Autodesk Inventor part; units mm, degrees
ref_plane "Start Plane" through (0, 0, 0) normal (0, 0, 1) x (1, 0, 0)
ref_plane "End Plane" through (0, 0, 100) normal (0, 0, 1) x (1, 0, 0)
ref_plane "YZ Plane" through (0, 0, 0) normal (1, 0, 0) x (0, 1, 0)
ref_plane "Start Plane" through (0, 0, 0) normal (0, 0, 1) x (1, 0, 0)
ref_plane "End Plane" through (0, 0, 100) normal (0, 0, 1) x (1, 0, 0)
sketch "Sketch2" plane through (0, 0, 0) normal (0, 0, 1) x (1, 0, 0)
  circle A0 centre (0, 0) radius 2.5
  circle A1 centre (0, 0) radius 4.2 construction
  line L0 (10, -10) -> (-10, -10) construction
  line L1 (-10, -10) -> (-10, 10) construction
  line L2 (-10, 10) -> (10, 10) construction
  line L3 (10, 10) -> (10, -10) construction
  line L4 (10, -10) -> (-10, 10) construction
  line L5 (-10, -10) -> (10, 10) construction
  line L6 (-4.1658, 3.1759) -> (-7.7464, 6.7565)
  line L7 (-10, 8.8) -> (-10, 3.95)
  line L8 (-10, 3.95) -> (-9.6, 3.95)
  line L9 (-9.6, 3.95) -> (-9.6, 3.2)
  line L10 (-9.6, 3.2) -> (-8.6, 3.2)
  line L11 (-8.6, 3.2) -> (-8.6, 6.4029)
  line L12 (-10, 0) -> (0, 0) construction
  line L13 (-8.8, 10) -> (-3.95, 10)
  line L14 (-3.95, 10) -> (-3.95, 9.6)
  line L15 (-3.95, 9.6) -> (-3.2, 9.6)
  line L16 (-3.2, 9.6) -> (-3.2, 8.6)
  line L17 (-3.2, 8.6) -> (-6.4029, 8.6)
  arc A2 (-8.8, 10) -> (-10, 8.8) centre (-8.8, 8.8) ccw
  arc A3 (-6.4029, 8.6) -> (-6.7565, 7.7464) centre (-6.4029, 8.1) ccw
  arc A4 (-7.7464, 6.7565) -> (-8.6, 6.4029) centre (-8.1, 6.4029) ccw
  arc A5 (-3.8668, 1.6394) -> (-4.2, 0) centre (0, 0) ccw
  arc A6 (-3.8668, 1.6394) -> (-4.1658, 3.1759) centre (-5.1558, 2.1859) ccw
  line L18 (-3.1759, 4.1658) -> (-6.7565, 7.7464)
  arc A7 (0, 4.2) -> (-1.6394, 3.8668) centre (0, 0) ccw
  arc A8 (-3.1759, 4.1658) -> (-1.6394, 3.8668) centre (-2.1859, 5.1558) ccw
  line L19 (-3.2, -9.6) -> (-3.2, -8.6)
  line L20 (-3.2, -8.6) -> (-6.4029, -8.6)
  line L21 (-8.8, -10) -> (-3.95, -10)
  arc A9 (-1.6394, -3.8668) -> (-3.1759, -4.1658) centre (-2.1859, -5.1558) ccw
  line L22 (-3.1759, -4.1658) -> (-6.7565, -7.7464)
  line L23 (0, -10) -> (0, 0) construction
  arc A10 (-4.1658, -3.1759) -> (-3.8668, -1.6394) centre (-5.1558, -2.1859) ccw
  line L24 (-4.1658, -3.1759) -> (-7.7464, -6.7565)
  line L25 (-3.95, -9.6) -> (-3.2, -9.6)
  line L26 (-3.95, -10) -> (-3.95, -9.6)
  arc A11 (-1.6394, -3.8668) -> (0, -4.2) centre (0, 0) ccw
  arc A12 (-4.2, 0) -> (-3.8668, -1.6394) centre (0, 0) ccw
  line L27 (-9.6, -3.95) -> (-9.6, -3.2)
  arc A13 (-6.7565, -7.7464) -> (-6.4029, -8.6) centre (-6.4029, -8.1) ccw
  arc A14 (-8.6, -6.4029) -> (-7.7464, -6.7565) centre (-8.1, -6.4029) ccw
  line L28 (-8.6, -3.2) -> (-8.6, -6.4029)
  line L29 (-9.6, -3.2) -> (-8.6, -3.2)
  line L30 (-10, -3.95) -> (-9.6, -3.95)
  line L31 (-10, -8.8) -> (-10, -3.95)
  arc A15 (-10, -8.8) -> (-8.8, -10) centre (-8.8, -8.8) ccw
  line L32 (9.6, -3.2) -> (8.6, -3.2)
  line L33 (8.6, -3.2) -> (8.6, -6.4029)
  line L34 (10, -8.8) -> (10, -3.95)
  arc A16 (3.8668, -1.6394) -> (4.1658, -3.1759) centre (5.1558, -2.1859) ccw
  line L35 (4.1658, -3.1759) -> (7.7464, -6.7565)
  line L36 (10, 0) -> (0, 0) construction
  arc A17 (3.1759, -4.1658) -> (1.6394, -3.8668) centre (2.1859, -5.1558) ccw
  line L37 (3.1759, -4.1658) -> (6.7565, -7.7464)
  line L38 (9.6, -3.95) -> (9.6, -3.2)
  line L39 (10, -3.95) -> (9.6, -3.95)
  arc A18 (3.8668, -1.6394) -> (4.2, 0) centre (0, 0) ccw
  arc A19 (0, -4.2) -> (1.6394, -3.8668) centre (0, 0) ccw
  line L40 (3.95, -9.6) -> (3.2, -9.6)
  arc A20 (7.7464, -6.7565) -> (8.6, -6.4029) centre (8.1, -6.4029) ccw
  arc A21 (6.4029, -8.6) -> (6.7565, -7.7464) centre (6.4029, -8.1) ccw
  line L41 (3.2, -8.6) -> (6.4029, -8.6)
  line L42 (3.2, -9.6) -> (3.2, -8.6)
  line L43 (3.95, -10) -> (3.95, -9.6)
  line L44 (8.8, -10) -> (3.95, -10)
  arc A22 (8.8, -10) -> (10, -8.8) centre (8.8, -8.8) ccw
  line L45 (3.2, 9.6) -> (3.2, 8.6)
  line L46 (3.2, 8.6) -> (6.4029, 8.6)
  line L47 (8.8, 10) -> (3.95, 10)
  arc A23 (1.6394, 3.8668) -> (3.1759, 4.1658) centre (2.1859, 5.1558) ccw
  line L48 (3.1759, 4.1658) -> (6.7565, 7.7464)
  line L49 (0, 10) -> (0, 0) construction
  arc A24 (4.1658, 3.1759) -> (3.8668, 1.6394) centre (5.1558, 2.1859) ccw
  line L50 (4.1658, 3.1759) -> (7.7464, 6.7565)
  line L51 (3.95, 9.6) -> (3.2, 9.6)
  line L52 (3.95, 10) -> (3.95, 9.6)
  arc A25 (1.6394, 3.8668) -> (0, 4.2) centre (0, 0) ccw
  arc A26 (4.2, 0) -> (3.8668, 1.6394) centre (0, 0) ccw
  line L53 (9.6, 3.95) -> (9.6, 3.2)
  arc A27 (6.7565, 7.7464) -> (6.4029, 8.6) centre (6.4029, 8.1) ccw
  arc A28 (8.6, 6.4029) -> (7.7464, 6.7565) centre (8.1, 6.4029) ccw
  line L54 (8.6, 3.2) -> (8.6, 6.4029)
  line L55 (9.6, 3.2) -> (8.6, 3.2)
  line L56 (10, 3.95) -> (9.6, 3.95)
  line L57 (10, 8.8) -> (10, 3.95)
  arc A29 (10, 8.8) -> (8.8, 10) centre (8.8, 8.8) ccw
  point P0 (-3.4233, 2.4333)
  point P1 (-8.6, 7.6101)
  point P2 (-7.6101, 8.6)
  point P3 (-7.6101, -8.6)
  point P4 (-10, -10)
  point P5 (-2.4333, -3.4233)
  point P6 (-8.6, -7.6101)
  point P7 (8.6, -7.6101)
  point P8 (10, -10)
  point P9 (3.4233, -2.4333)
  point P10 (7.6101, -8.6)
  point P11 (7.6101, 8.6)
  point P12 (10, 10)
  point P13 (2.4333, 3.4233)
  point P14 (8.6, 7.6101)
  point P15 (-4.2, 0)
  point P16 (0, -4.2)
  point P17 (4.2, 0)
  point P18 (0, 4.2)
  dimension "d8" = 5
  dimension "d9" = 8.4
  dimension "d10" = 20
  dimension "d11" = 20
  dimension "d13" = 1.4
  dimension "d14" = 3.2
  dimension "d15" = 3.95
  dimension "d16" = 0.4
  dimension "d18" = 1.2
  dimension "d19" = 0.5
  dimension "d20" = 1.4
  dimension "d21" = 1.4
  dimension "d24" = 360
extrude "Body" add sketch "Sketch2" along normal up to surface (100 mm away) from surface at 0
sketch "Sketch11" plane through (0, 0, 0) normal (0, 0, 1) x (1, 0, 0)
  line L0 (0, 0) -> (10, 0)
ref_plane "Work Plane11" through (0, 0, 0) normal (0, -1, 0) x (1, 0, 0)
sketch "Sketch12" plane through (0, 0, 0) normal (0, -1, 0) x (1, 0, 0)
  line L0 (-14, 0) -> (14, 0)
  line L1 (-14, 100) -> (14, 100)
  dimension "d53" = 100
equation "\"G_OFFSET_START\" = 0"
equation "\"G_OFFSET_END\" = 0"
equation "\"G_L\" = d53"
equation "\"G_OFFSET_START1\" = 0"
equation "\"G_OFFSET_END1\" = 0"
equation "\"G_OFFSET_START2\" = 0"
equation "\"G_OFFSET_END2\" = 0"
properties part number "2020Profile" material "Aluminum 6061"
Source: CAD feature listing. Evaluate the final solid. Frame: model axes, mm. A direction names the side the tool comes from. Give positions to 0.01 mm unless a question says otherwise; leave off trailing zeros. Use a Markdown table: item, result. Add a question column.
1) Reachability of faces 1 (the face through (0.848, -4.113, 49.3)), 2 (the face through (4.12, -0.82, 49.3)), 3 (the face through (-4.12, 0.82, 49.3)), 4 (the face through (8.6, 5, 49)), 5 (the face through (-6, -10, 49)) from +Z, -Z, +X, -X, +Y, -Y: full face, straight path, thin tool, end or side. Return the list, or none.
2) Line query: line 1 along X through (y, z) = (-8, 76); line 2 along Y through (x, z) = (-5, 49); line 3 along Y through (x, z) = (0, 69). Output: solid intervals per line, ascending. Write a range as [from, to].
3) First-contact query: pin 1 (2 mm diameter, centred on x = 1.5, z = 76, fed in from -Y); pin 2 (1.5 mm diameter, centred on y = -2.5, z = 31, fed in from +X); pin 3 (0.8 mm diameter, centred on x = 3.5, z = 68.5, fed in from -Y). Flat tips, straight axial feed; report the tip coordinate or a pass-through.
4) Pull-direction query (X, two-part tool) for faces 6 (the face through (4.113, 0.848, 49.3)), 7 (the face through (6, 10, 49)), 8 (the face through (-5, -8.6, 49)); classes: +X half, -X half, draft (parallel to the pull), parting line (faces both ways), or undercut.
Numbers:
| question | item | result |
|---|---|---|
| 1 | face 1 | +Z, -Z, -Y |
| 1 | face 2 | +Z, -Z, +X |
| 1 | face 3 | +Z, -Z, -X |
| 1 | face 4 | +Z, -Z |
| 1 | face 5 | +Z, -Z, +X, -X, -Y |
| 2 | line 1 | x = [-10, -6.89], [6.89, 10] |
| 2 | line 2 | y = [-10, -8.6], [-5.99, -4.01], [4.01, 5.99], [8.6, 10] |
| 2 | line 3 | y = [-4.2, -2.5], [2.5, 4.2] |
| 3 | pin 1 | stops at y = -4.17 |
| 3 | pin 2 | stops at x = 9.6 |
| 3 | pin 3 | stops at y = -9.6 |
| 4 | face 6 | +X half |
| 4 | face 7 | draft |
| 4 | face 8 | undercut |
